Here's how the part is built. I have some questions about the finished solid (model axes, mm). A direction names the side the tool comes from. Round coordinates to 2 decimals unless told otherwise and drop trailing zeros. Write each loop counter-clockwise with the first axis right and the second up, starting at its lowest first coordinate (ties: lowest second). Pieces come first, ordered by that corner, then holes. Notation, with made-up numbers: M 72.25,37 L 106.25,37 A28 cw 106.25,68 Z; hole C 74,76.5 d7. An arc over 180 degrees is marked long. Use a Markdown table: item, result. Add a question column.
```python
from build123d import *

# Parameters (mm, degrees)
F3_DEPTH = 1
F4_R     = 5


with BuildPart() as f1:
    # F0 (on Front) → F1 (revolve)
    with BuildSketch(Plane.XZ):
        with BuildLine():
            Line((5.5, 0), (6, 0))
            ThreePointArc((6, 0), (4.2426406871, 4.2426406871), (0, 6))
            Line((0, 6), (0, 5.5))
            ThreePointArc((0, 5.5), (1.2856151892, 5.3476343915), (2.5, 4.8989794856))
            ThreePointArc((2.5, 4.8989794856), (3.0178958157, 4.5980762114), (3.5, 4.2426406871))
            ThreePointArc((3.5, 4.2426406871), (4.9749371855, 2.3452078799), (5.5, 0))
        make_face()
        with BuildLine():
            Line((3.5, 2.5), (3.5, 4.2426406871))
            ThreePointArc((3.5, 4.2426406871), (3.0178958157, 4.5980762114), (2.5, 4.8989794856))
            Line((2.5, 4.8989794856), (2.5, 2.5))
            Line((2.5, 2.5), (3.5, 2.5))
        make_face()
    revolve(axis=Axis((0, 0, 3), (0, 0, -1)))

    # F2 (on face) → F3 (join)
    with BuildSketch(Plane(origin=(0, 0, 0), x_dir=(1, 0, 0), z_dir=(0, 0, -1))):
        with BuildLine():
            Line((-6.0000796802, 5), (-6.0000796802, 0))
            Line((-6.0000796802, 0), (-5.5000796802, 0))
            ThreePointArc((-5.5000796802, 0), (0, 5.4891055059), (5.5000796802, 0))
            Line((5.5000796802, 0), (6.0000796802, 0))
            Line((6.0000796802, 0), (6.0000796802, 5))
            ThreePointArc((6.0000796802, 5), (0, 8.9616150573), (-6.0000796802, 5))
        make_face()
    extrude(amount=-F3_DEPTH)

    # F4
    f4_edges = [f1.edges().sort_by_distance(p)[0] for p in [
        (6.00008, -5, 0.5),
        (-6.00008, -5, 0.5),
    ]]
    fillet(f4_edges, radius=F4_R)


solid = f1.part
```
Item 1: Imagine slicing it at D-D on z = 2. List the corners of the cut face in (x, y) for me.
Item 2: For pin 1 Ø2 at (y, z) = (-3, 3.5) entering from -X; pin 2 Ø1.5 at (x, y) = (-2.5, 0) entering from -Z; pin 3 Ø1 at (x, y) = (-1, 3.5) entering from +Z, each with a flat end and sliding along its axis, tell me the tip position at first contact or that it passes through.
Item 3: I need wall thicknesses on probe 1 along X at (y, z) = (0, 3.35); probe 2 along X at (y, z) = (0, 3.8); probe 3 along Y at (x, z) = (0.5, 3). Which ranges of each line are inside material? Lowest first, please. Write a range as from..to.
Item 4: If we mould it in two halves opening along Y, with no side actions, what happens to faces 1 (the face through (0.07, -8.96, 0.49)), 2 (the face through (0, -6, 0)), 3 (the face through (3.233, 1.341, 3.384))? For each: +Y half, -Y half, draft (parallel to the pull), parting line (faces both ways), or undercut.
Item 5: On a 3-axis mill with a long thin cutter (end or side, diameter ignored), from which of +Z, -Z, +X, -X, +Y, -Y can I reach the whole of each face in a straight line? I mean faces 4 (the face through (-6, -1.8, 0.5)), 5 (the face through (-2, 2, 2.5)), 6 (the face through (0, -6.5, 1)). Say none if no direction works.
Item 6: Imagine slicing it at A-A on x = 0. List the corners of the cut face in (y, z) for me.
Item 7: Imagine slicing it at B-B on y = -1.25. List the corners of the cut face in (x, z) for me.
Item 8: Imagine slicing it at C-C on z = 3.5. List the corners of the cut face in (x, y) for me, plus the area to 3 significant figures.
The answers:
| question | item | result |
|---|---|---|
| 1 | outline | C 0,0 d11.31; hole C 0,0 d10.25 |
| 2 | pin 1 | x = -4.79 |
| 2 | pin 2 | z = 2.5 |
| 2 | pin 3 | z = 5.11 |
| 3 | probe 1 | -4.98..-4.36, -3.5..-2.5, 2.5..3.5, 4.36..4.98 |
| 3 | probe 2 | -4.64..-3.98, -3.5..-2.5, 2.5..3.5, 3.98..4.64 |
| 3 | probe 3 | -5.17..-4.58, -3.46..-2.45, 2.45..3.46, 4.58..5.17 |
| 4 | face 1 | -Y half |
| 4 | face 2 | draft |
| 4 | face 3 | undercut |
| 5 | face 4 | +Z, -Z, -X, +Y, -Y |
| 5 | face 5 | -Z |
| 5 | face 6 | +Z, -Y |
| 6 | outline | M -8.96,0 L -5.49,0 L -5.49,0.35 A5.5 cw -3.5,4.24 L -3.5,2.5 L -2.5,2.5 L -2.5,4.9 A5.5 cw 2.5,4.9 L 2.5,2.5 L 3.5,2.5 L 3.5,4.24 A5.5 cw 5.5,0 L 6,0 A6 ccw -5.92,1 L -8.96,1 Z |
| 7 | outline | M -6,0 L -5.35,0 L -5.35,0.16 A5.36 cw -3.27,4.24 L -3.27,2.5 L -2.17,2.5 L -2.17,4.9 A5.36 cw 2.17,4.9 L 2.17,2.5 L 3.27,2.5 L 3.27,4.24 A5.36 cw 5.35,0.16 L 5.35,0 L 6,0 L 6,1 L 5.78,1 A5.87 ccw -5.78,1 L -6,1 Z |
| 8 | outline | C 0,0 d9.75; C 0,0 d7; hole C 0,0 d8.49; hole C 0,0 d5 |
| 8 | area | 36.9 mm² |
